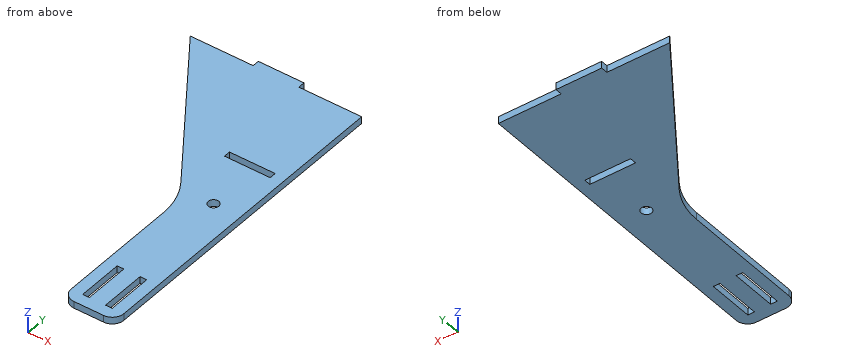
from build123d import *

# Parameters (mm, degrees)
SKETCH1_W           = 2.9
SKETCH1_H           = 20
BOSS_EXTRUDE1_DEPTH = 3
FILLET1_R           = 5
FILLET2_R           = 30
SKETCH4_R           = 2.3
CUT_EXTRUDE1_DEPTH  = 10
SKETCH5_W           = 20
SKETCH5_H           = 2.9
CUT_EXTRUDE2_DEPTH  = 4


with BuildPart() as part:
    # Sketch1 → Boss-Extrude1 (new body)
    with BuildSketch(Plane.XY):
        Polygon((0, 0), (-23, 0), (-23, 68), (-75, 143), (-47.5, 143), (-47.5, 146), (-27.5, 146), (-27.5, 143), (0, 143), align=None)
        with Locations((-16.5, 15)):
            Rectangle(SKETCH1_W, SKETCH1_H, mode=Mode.SUBTRACT)
        with Locations((-6.5, 15)):
            Rectangle(SKETCH1_W, SKETCH1_H, mode=Mode.SUBTRACT)
    extrude(amount=BOSS_EXTRUDE1_DEPTH)

    # Fillet1
    fillet1_edges = [part.edges().sort_by_distance(p)[0] for p in [
        (0, 0, 1.5),
        (-23, 0, 1.5),
    ]]
    fillet(fillet1_edges, radius=FILLET1_R)

    # Fillet2
    fillet2_edges = [part.edges().sort_by_distance(p)[0] for p in [
        (-23, 68, 1.5),
    ]]
    fillet(fillet2_edges, radius=FILLET2_R)

    # Sketch4 → Cut-Extrude1 (cut)
    with BuildSketch(Plane.XY.offset(3)):
        with Locations((-12, 73)):
            Circle(SKETCH4_R)
    extrude(amount=-CUT_EXTRUDE1_DEPTH, mode=Mode.SUBTRACT)

    # Sketch5 → Cut-Extrude2 (cut, through all)
    with BuildSketch(Plane(origin=(0, 0, 0), x_dir=(-1, 0, 0), z_dir=(0, 0, -1))):
        with Locations((15, 98)):
            Rectangle(SKETCH5_W, SKETCH5_H)
    extrude(amount=-CUT_EXTRUDE2_DEPTH, mode=Mode.SUBTRACT)


solid = part.part
Model file for the job. Use its own axes, mm. Give positions to 0.01 mm unless a question says otherwise; leave off trailing zeros. Loops run counter-clockwise (first coordinate to the right, second up) from the corner with the lowest first, then second, coordinate; pieces in that order, holes last.
Item 1: Slice it at B-B (y = 73). Write the cut outline in (x, z).
Check values:
outline: (-26.67, 0) - (-14.3, 0) - (-14.3, 3) - (-26.67, 3) - close; (-9.7, 0) - (0, 0) - (0, 3) - (-9.7, 3) - close
Item 2: Slice it at C-C (z = 2.2). Write the cut outline in (x, y), plus the area to 3 significant figures.
Check values:
outline: (-75, 143) - (-28.35, 75.71) arc R30 cw to (-23, 58.62) - (-23, 5) arc R5 ccw to (-18, 0) - (-5, 0) arc R5 ccw to (0, 5) - (0, 143) - (-27.5, 143) - (-27.5, 146) - (-47.5, 146) - (-47.5, 143) - close; hole (-25, 96.55) - (-5, 96.55) - (-5, 99.45) - (-25, 99.45) - close; hole (-17.95, 5) - (-15.05, 5) - (-15.05, 25) - (-17.95, 25) - close; hole circle Ø4.6 at (-12, 73); hole (-7.95, 5) - (-5.05, 5) - (-5.05, 25) - (-7.95, 25) - close
area: 5,110 mm2
Item 3: Slice it at A-A (x = -12). Write the cut outline in (y, z), plus the area to 4 significant figures.
Check values:
outline: (0, 0) - (70.7, 0) - (70.7, 3) - (0, 3) - close; (75.3, 0) - (96.55, 0) - (96.55, 3) - (75.3, 3) - close; (99.45, 0) - (143, 0) - (143, 3) - (99.45, 3) - close
area: 406.5 mm2
Item 4: Drop a flat-ended pin along its axis: P1, Ø1.5, axis at x = -67, z = 1, coming from the +Y side. Give the stop position or say it passes through.
Check values:
P1: stops at y = 143
Item 5: Slice it at D-D (y = 136). Write the cut outline in (x, z).
Check values:
outline: (-70.15, 0) - (0, 0) - (0, 3) - (-70.15, 3) - close
Item 6: Drill centre lines: line 1 along Y through (x, z) = (-12, 2.3); line 2 along X through (y, z) = (97, 0.3); line 3 along X through (y, z) = (28, 1.7). Where is each one in solid material? Low to high.
Check values:
line 1: y = 0 to 70.7, 75.3 to 96.55, 99.45 to 143
line 2: x = -43.11 to -25, -5 to 0
line 3: x = -23 to 0
